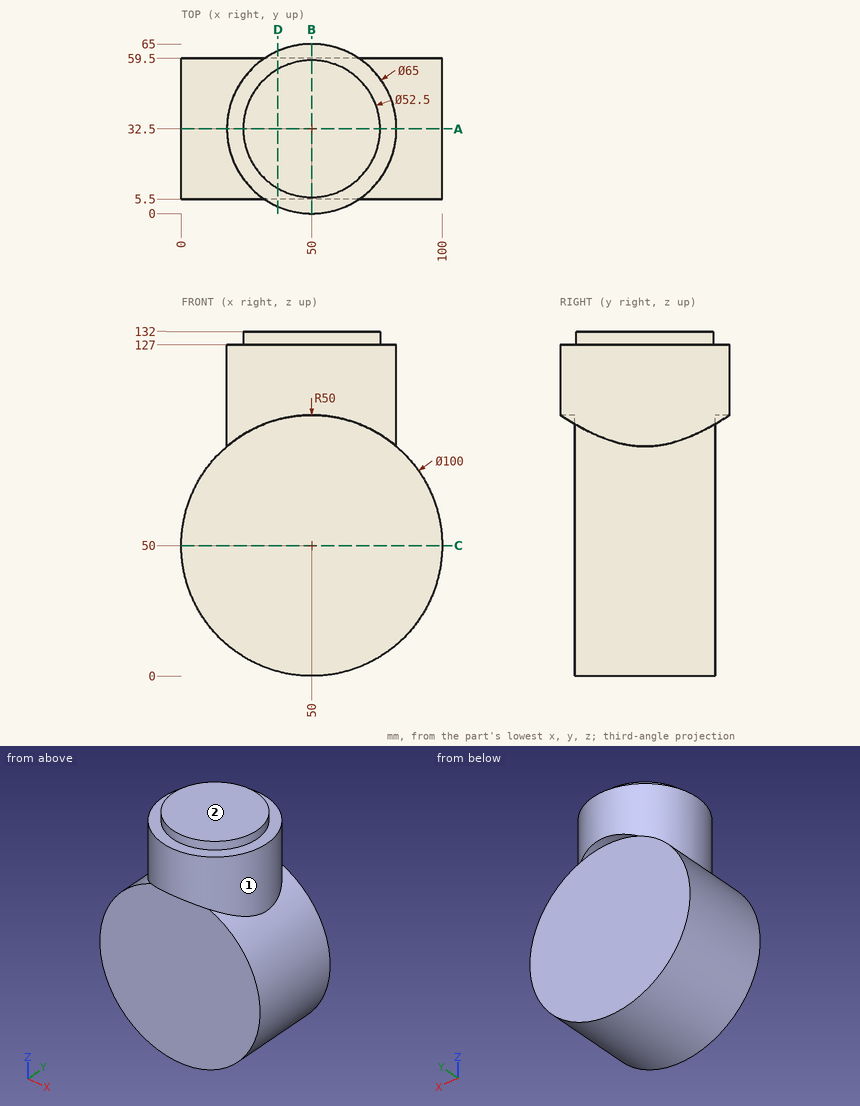
Could you check a few things on this drawing? It's one solid part, dimensions in mm from its lowest x, y, z. A direction names the side the tool comes from. Round coordinates to 2 decimals unless told otherwise and drop trailing zeros. Order: outer loops, then holes, each group sorted by start corner. A loop starts at its lowest first (then second) coordinate and runs counter-clockwise, first axis right, second up.
Q1. Imagine slicing it at D-D, the plane x = 37. List the corners of the cut face in (y, z) for me.
Geometry says:
outline: (2.71, 98.28) - (5.5, 98.28) - (5.5, 1.72) - (59.5, 1.72) - (59.5, 98.28) - (62.29, 98.28) - (62.29, 127) - (55.3, 127) - (55.3, 132) - (9.7, 132) - (9.7, 127) - (2.71, 127) - close
Q2. Imagine slicing it at C-C, the plane z = 50. List the corners of the cut face in (x, y) for me, then the cut area to 3 significant figures.
Geometry says:
outline: (0, 5.5) - (100, 5.5) - (100, 59.5) - (0, 59.5) - close
area: 5,400 mm2
Q3. Imagine slicing it at A-A, the plane y = 32.5. List the corners of the cut face in (x, z) for me, then the cut area to 3 significant figures.
Geometry says:
outline: (17.5, 88) arc R50 ccw (long way) to (82.5, 88) - (82.5, 127) - (76.25, 127) - (76.25, 132) - (23.75, 132) - (23.75, 127) - (17.5, 127) - close
area: 10,100 mm2
Q4. Imagine slicing it at B-B, the plane x = 50. List the corners of the cut face in (y, z) for me.
Geometry says:
outline: (0, 100) - (5.5, 100) - (5.5, 0) - (59.5, 0) - (59.5, 100) - (65, 100) - (65, 127) - (58.75, 127) - (58.75, 132) - (6.25, 132) - (6.25, 127) - (0, 127) - close
Q5. Which directions (+Z, -Z, +X, -X, +Y, -Y) give clear straight access to the entire face, cutting with the end or side of a thin tool? Please do the marked faces 1 and 2.
Geometry says:
face 1: +Z
face 2: +Z, +X, -X, +Y, -Y
Q6. Please list where these lines run through material, in increasing order: probe 1 along Y at (x, z) = (63, 45.5); probe 2 along Z at (x, y) = (50.5, 54); probe 3 along X at (y, z) = (48.5, 29).
Geometry says:
probe 1: y = 5.5 to 59.5
probe 2: z = 0 to 132
probe 3: x = 4.62 to 95.38
Q7. I'm going to push flat-ended pins straight in: P1, Ø1, axis at y = 13.5, z = 76.5, coming from the -X side; P2, Ø8, axis at y = 15, z = 79, coming from the -X side; P3, Ø3, axis at x = 26, y = 57, coming from the +Z side. Where does each tip first touch, or does it pass through?
Geometry says:
P1: stops at x = 7.29
P2: stops at x = 6.7
P3: stops at z = 94.65
